```python
from build123d import *

# Parameters (mm, degrees)
F1_DEPTH = 19.05
F2_R     = 1.6880243077
F3_DEPTH = 19.05
F4_DEPTH = 19.05


with BuildPart() as f1:
    # F0 (on Front) → F1 (new body)
    with BuildSketch(Plane.XZ):
        with BuildLine():
            ThreePointArc((15.778162915, -1.0689673082), (15.8052876039, -0.5347895271), (15.8143326157, 0))
            ThreePointArc((15.8143326157, 0), (15.8010341981, 0.6484090916), (15.7611613108, 1.2957276769))
            ThreePointArc((15.7611613108, 1.2957276769), (15.0048006195, 4.9949048489), (13.3931251572, 8.4093587509))
            ThreePointArc((13.3931251572, 8.4093587509), (12.7269029213, 9.3871751934), (11.9894377321, 10.3124438882))
            ThreePointArc((11.9894377321, 10.3124438882), (9.2032072916, 12.8605634257), (5.8923688049, 14.6755955908))
            ThreePointArc((5.8923688049, 14.6755955908), (4.7786376097, 15.0750701051), (3.6381564457, 15.3901570413))
            ThreePointArc((3.6381564457, 15.3901570413), (-0.1136984162, 15.8139238884), (-3.8590721566, 15.3362537202))
            ThreePointArc((-3.8590721566, 15.3362537202), (-4.9949048489, 15.0048006195), (-6.1027769466, 14.5893532968))
            ThreePointArc((-6.1027769466, 14.5893532968), (-9.3871751934, 12.7269029213), (-12.1364787193, 10.1389841885))
            ThreePointArc((-12.1364787193, 10.1389841885), (-12.8605634257, 9.2032072916), (-13.512656971, 8.2159124668))
            ThreePointArc((-13.512656971, 8.2159124668), (-15.0750701051, 4.7786376097), (-15.778162915, 1.0689673082))
            ThreePointArc((-15.778162915, 1.0689673082), (-15.8139238884, -0.1136984162), (-15.7611613108, -1.2957276769))
            ThreePointArc((-15.7611613108, -1.2957276769), (-15.0048006195, -4.9949048489), (-13.3931251572, -8.4093587509))
            ThreePointArc((-13.3931251572, -8.4093587509), (-12.7269029213, -9.3871751934), (-11.9894377321, -10.3124438882))
            ThreePointArc((-11.9894377321, -10.3124438882), (-9.2032072916, -12.8605634257), (-5.8923688049, -14.6755955908))
            ThreePointArc((-5.8923688049, -14.6755955908), (-4.7786376097, -15.0750701051), (-3.6381564457, -15.3901570413))
            ThreePointArc((-3.6381564457, -15.3901570413), (0.1136984162, -15.8139238884), (3.8590721566, -15.3362537202))
            ThreePointArc((3.8590721566, -15.3362537202), (4.9949048489, -15.0048006195), (6.1027769466, -14.5893532968))
            ThreePointArc((6.1027769466, -14.5893532968), (9.3871751934, -12.7269029213), (12.1364787193, -10.1389841885))
            ThreePointArc((12.1364787193, -10.1389841885), (12.8605634257, -9.2032072916), (13.512656971, -8.2159124668))
            ThreePointArc((13.512656971, -8.2159124668), (15.0750701051, -4.7786376097), (15.778162915, -1.0689673082))
        make_face()
    extrude(amount=F1_DEPTH)

    # F2 (on face) → F3 (cut)
    with BuildSketch(Plane.XZ.offset(19.05)):
        Circle(F2_R)
    extrude(amount=-F3_DEPTH, mode=Mode.SUBTRACT)

    # F0 (on Front) → F4 (join)
    with BuildSketch(Plane.XZ):
        with BuildLine():
            ThreePointArc((15.7611613108, 1.2957276769), (15.8010341981, 0.6484090916), (15.8143326157, 0))
            ThreePointArc((15.8143326157, 0), (15.8052876039, -0.5347895271), (15.778162915, -1.0689673082))
            Line((15.778162915, -1.0689673082), (17.2791990232, 0.0449688409))
            Line((17.2791990232, 0.0449688409), (15.7611613108, 1.2957276769))
        make_face()
        with BuildLine():
            ThreePointArc((13.3931251572, 8.4093587509), (15.0048006195, 4.9949048489), (15.7611613108, 1.2957276769))
            Line((15.7611613108, 1.2957276769), (17.2791990232, 0.0449688409))
            Line((17.2791990232, 0.0449688409), (22.4461490806, 3.8794218687))
            Line((22.4461490806, 3.8794218687), (19.6925609503, 6.2533739679))
            Line((19.6925609503, 6.2533739679), (20.5248865096, 9.7924600538))
            Line((20.5248865096, 9.7924600538), (13.9527336374, 10.1928389138))
            Line((13.9527336374, 10.1928389138), (13.3931251572, 8.4093587509))
        make_face()
        with BuildLine():
            Line((17.2791990232, 0.0449688409), (15.778162915, -1.0689673082))
            ThreePointArc((15.778162915, -1.0689673082), (15.0750701051, -4.7786376097), (13.512656971, -8.2159124668))
            Line((13.512656971, -8.2159124668), (14.0055976804, -10.1200778007))
            Line((14.0055976804, -10.1200778007), (20.4395830263, -10.0549971802))
            Line((20.4395830263, -10.0549971802), (19.6072574669, -6.5159110943))
            Line((19.6072574669, -6.5159110943), (22.3608455972, -4.1419589951))
            Line((22.3608455972, -4.1419589951), (17.2791990232, 0.0449688409))
        make_face()
        with BuildLine():
            ThreePointArc((11.9894377321, 10.3124438882), (12.7269029213, 9.3871751934), (13.3931251572, 8.4093587509))
            Line((13.3931251572, 8.4093587509), (13.9527336374, 10.1928389138))
            Line((13.9527336374, 10.1928389138), (11.9894377321, 10.3124438882))
        make_face()
        with BuildLine():
            Line((14.0055976804, -10.1200778007), (13.512656971, -8.2159124668))
            ThreePointArc((13.512656971, -8.2159124668), (12.8605634257, -9.2032072916), (12.1364787193, -10.1389841885))
            Line((12.1364787193, -10.1389841885), (14.0055976804, -10.1200778007))
        make_face()
        with BuildLine():
            ThreePointArc((5.8923688049, 14.6755955908), (9.2032072916, 12.8605634257), (11.9894377321, 10.3124438882))
            Line((11.9894377321, 10.3124438882), (13.9527336374, 10.1928389138))
            Line((13.9527336374, 10.1928389138), (15.8790491026, 16.3320336204))
            Line((15.8790491026, 16.3320336204), (12.2559754761, 16.6340827186))
            Line((12.2559754761, 16.6340827186), (10.8491183906, 19.9864921956))
            Line((10.8491183906, 19.9864921956), (5.2967982382, 16.4473909634))
            Line((5.2967982382, 16.4473909634), (5.8923688049, 14.6755955908))
        make_face()
        with BuildLine():
            Line((14.0055976804, -10.1200778007), (12.1364787193, -10.1389841885))
            ThreePointArc((12.1364787193, -10.1389841885), (9.3871751934, -12.7269029213), (6.1027769466, -14.5893532968))
            Line((6.1027769466, -14.5893532968), (5.3823340565, -16.4195986913))
            Line((5.3823340565, -16.4195986913), (10.6257909718, -20.148749063))
            Line((10.6257909718, -20.148749063), (12.0326480574, -16.796339586))
            Line((12.0326480574, -16.796339586), (15.6557216838, -16.4942904878))
            Line((15.6557216838, -16.4942904878), (14.0055976804, -10.1200778007))
        make_face()
        with BuildLine():
            ThreePointArc((3.6381564457, 15.3901570413), (4.7786376097, 15.0750701051), (5.8923688049, 14.6755955908))
            Line((5.8923688049, 14.6755955908), (5.2967982382, 16.4473909634))
            Line((5.2967982382, 16.4473909634), (3.6381564457, 15.3901570413))
        make_face()
        with BuildLine():
            Line((5.3823340565, -16.4195986913), (6.1027769466, -14.5893532968))
            ThreePointArc((6.1027769466, -14.5893532968), (4.9949048489, -15.0048006195), (3.8590721566, -15.3362537202))
            Line((3.8590721566, -15.3362537202), (5.3823340565, -16.4195986913))
        make_face()
        with BuildLine():
            ThreePointArc((-3.8590721566, 15.3362537202), (-0.1136984162, 15.8139238884), (3.6381564457, 15.3901570413))
            Line((3.6381564457, 15.3901570413), (5.2967982382, 16.4473909634))
            Line((5.2967982382, 16.4473909634), (3.2466920765, 22.5463636346))
            Line((3.2466920765, 22.5463636346), (0.1380239354, 20.6611372425))
            Line((0.1380239354, 20.6611372425), (-2.9706442056, 22.5463636346))
            Line((-2.9706442056, 22.5463636346), (-5.3823340565, 16.4195986913))
            Line((-5.3823340565, 16.4195986913), (-3.8590721566, 15.3362537202))
        make_face()
        with BuildLine():
            Line((5.3823340565, -16.4195986913), (3.8590721566, -15.3362537202))
            ThreePointArc((3.8590721566, -15.3362537202), (0.1136984162, -15.8139238884), (-3.6381564457, -15.3901570413))
            Line((-3.6381564457, -15.3901570413), (-5.2967982382, -16.4473909634))
            Line((-5.2967982382, -16.4473909634), (-3.2466920765, -22.5463636346))
            Line((-3.2466920765, -22.5463636346), (-0.1380239354, -20.6611372425))
            Line((-0.1380239354, -20.6611372425), (2.9706442056, -22.5463636346))
            Line((2.9706442056, -22.5463636346), (5.3823340565, -16.4195986913))
        make_face()
        with BuildLine():
            ThreePointArc((-6.1027769466, 14.5893532968), (-4.9949048489, 15.0048006195), (-3.8590721566, 15.3362537202))
            Line((-3.8590721566, 15.3362537202), (-5.3823340565, 16.4195986913))
            Line((-5.3823340565, 16.4195986913), (-6.1027769466, 14.5893532968))
        make_face()
        with BuildLine():
            Line((-5.2967982382, -16.4473909634), (-3.6381564457, -15.3901570413))
            ThreePointArc((-3.6381564457, -15.3901570413), (-4.7786376097, -15.0750701051), (-5.8923688049, -14.6755955908))
            Line((-5.8923688049, -14.6755955908), (-5.2967982382, -16.4473909634))
        make_face()
        with BuildLine():
            ThreePointArc((-12.1364787193, 10.1389841885), (-9.3871751934, 12.7269029213), (-6.1027769466, 14.5893532968))
            Line((-6.1027769466, 14.5893532968), (-5.3823340565, 16.4195986913))
            Line((-5.3823340565, 16.4195986913), (-10.6257909718, 20.148749063))
            Line((-10.6257909718, 20.148749063), (-12.0326480574, 16.796339586))
            Line((-12.0326480574, 16.796339586), (-15.6557216838, 16.4942904878))
            Line((-15.6557216838, 16.4942904878), (-14.0055976804, 10.1200778007))
            Line((-14.0055976804, 10.1200778007), (-12.1364787193, 10.1389841885))
        make_face()
        with BuildLine():
            Line((-5.2967982382, -16.4473909634), (-5.8923688049, -14.6755955908))
            ThreePointArc((-5.8923688049, -14.6755955908), (-9.2032072916, -12.8605634257), (-11.9894377321, -10.3124438882))
            Line((-11.9894377321, -10.3124438882), (-13.9527336374, -10.1928389138))
            Line((-13.9527336374, -10.1928389138), (-15.8790491026, -16.3320336204))
            Line((-15.8790491026, -16.3320336204), (-12.2559754761, -16.6340827186))
            Line((-12.2559754761, -16.6340827186), (-10.8491183906, -19.9864921956))
            Line((-10.8491183906, -19.9864921956), (-5.2967982382, -16.4473909634))
        make_face()
        with BuildLine():
            ThreePointArc((-13.512656971, 8.2159124668), (-12.8605634257, 9.2032072916), (-12.1364787193, 10.1389841885))
            Line((-12.1364787193, 10.1389841885), (-14.0055976804, 10.1200778007))
            Line((-14.0055976804, 10.1200778007), (-13.512656971, 8.2159124668))
        make_face()
        with BuildLine():
            Line((-13.9527336374, -10.1928389138), (-11.9894377321, -10.3124438882))
            ThreePointArc((-11.9894377321, -10.3124438882), (-12.7269029213, -9.3871751934), (-13.3931251572, -8.4093587509))
            Line((-13.3931251572, -8.4093587509), (-13.9527336374, -10.1928389138))
        make_face()
        with BuildLine():
            ThreePointArc((-15.778162915, 1.0689673082), (-15.0750701051, 4.7786376097), (-13.512656971, 8.2159124668))
            Line((-13.512656971, 8.2159124668), (-14.0055976804, 10.1200778007))
            Line((-14.0055976804, 10.1200778007), (-20.4395830263, 10.0549971802))
            Line((-20.4395830263, 10.0549971802), (-19.6072574669, 6.5159110943))
            Line((-19.6072574669, 6.5159110943), (-22.3608455972, 4.1419589951))
            Line((-22.3608455972, 4.1419589951), (-17.2791990232, -0.0449688409))
            Line((-17.2791990232, -0.0449688409), (-15.778162915, 1.0689673082))
        make_face()
        with BuildLine():
            Line((-13.9527336374, -10.1928389138), (-13.3931251572, -8.4093587509))
            ThreePointArc((-13.3931251572, -8.4093587509), (-15.0048006195, -4.9949048489), (-15.7611613108, -1.2957276769))
            Line((-15.7611613108, -1.2957276769), (-17.2791990232, -0.0449688409))
            Line((-17.2791990232, -0.0449688409), (-22.4461490806, -3.8794218687))
            Line((-22.4461490806, -3.8794218687), (-19.6925609503, -6.2533739679))
            Line((-19.6925609503, -6.2533739679), (-20.5248865096, -9.7924600538))
            Line((-20.5248865096, -9.7924600538), (-13.9527336374, -10.1928389138))
        make_face()
        with BuildLine():
            ThreePointArc((-15.7611613108, -1.2957276769), (-15.8139238884, -0.1136984162), (-15.778162915, 1.0689673082))
            Line((-15.778162915, 1.0689673082), (-17.2791990232, -0.0449688409))
            Line((-17.2791990232, -0.0449688409), (-15.7611613108, -1.2957276769))
        make_face()
    extrude(amount=F4_DEPTH)


solid = f1.part
```
Geometry check sheet. Reference: the model listing, model coordinates, mm. A direction names the side the tool comes from. Give positions to 0.01 mm unless a question says otherwise; leave off trailing zeros. Order: outer loops, then holes, each group sorted by start corner. A loop starts at its lowest first (then second) coordinate and runs counter-clockwise, first axis right, second up.
1. Gauge pin test, flat ends, axial feed: pin 1 Ø5 at (y, z) = (-17, -14) entering from -X; pin 2 Ø5 at (y, z) = (-6.5, 12) entering from -X; pin 3 Ø10 at (x, y) = (1, -4.5) entering from +Z; pin 4 Ø2 at (x, z) = (0, 0) entering from +Y. Record the tip position at first contact, or that the pin passes through.
2. Release check for a two-part mould opening along Z. For faces 5 (the face through (11.56, -9.39, 18.29)), 6 (the face through (19.83, -9.39, 1.94)), 7 (the face through (-11.56, -9.39, -18.29)) record: pulls with the +Z half, pulls with the -Z half, needs draft (parallel to the pull), parting line crosses it, or undercut.
3. Access from +Z, -Z, +X, -X, +Y, -Y to the whole of each face (thin tool, end or side, straight path). Record for faces 1 (the face through (17.28, -9.39, 9.99)), 2 (the face through (1.714, -9.392, 21.617)), 3 (the face through (-8.11, -9.39, -18.24)), 4 (the face through (-17.28, -9.39, -9.99)).
4. Thickness scan on L1, parallel to X at y = -4.75, z = 17.5; L2, parallel to X at y = -16.75, z = -1; L3, parallel to Z at x = 0, y = -6.5. Record the ranges inside material, lowest first.
5. Section check C-C, the plane z = -12.5. Enter the section's corners in (x, y).
6. Section check B-B, the plane x = -9. Enter the section's corners in (y, z).
7. Section check A-A, the plane x = -15. Enter the section's corners in (y, z), and give its area (3 significant figures).
Values follow:
1. pin 1: stops at x = -15.88
1. pin 2: stops at x = -20.44
1. pin 3: stops at z = 22.55
1. pin 4: passes through
2. face 5: pulls with the +Z half
2. face 6: undercut
2. face 7: pulls with the -Z half
3. face 1: +X, +Y, -Y
3. face 2: +Z, +Y, -Y
3. face 3: -Z, +Y, -Y
3. face 4: -X, +Y, -Y
4. L1: x = -11.74 to -6.9, -4.96 to 4.94, 6.95 to 11.89
4. L2: x = -18.57 to -1.36, 1.36 to 18.55
4. L3: z = -20.74 to -1.69, 1.69 to 20.74
5. outline: (-14.68, -19.05) - (14.62, -19.05) - (14.62, 0) - (-14.68, 0) - close
6. outline: (-19.05, -18.81) - (0, -18.81) - (0, 18.99) - (-19.05, 18.99) - close
7. outline: (-19.05, -16.41) - (0, -16.41) - (0, -13.53) - (-19.05, -13.53) - close; (-19.05, -10.13) - (0, -10.13) - (0, 10.11) - (-19.05, 10.11) - close; (-19.05, 13.96) - (0, 13.96) - (0, 16.55) - (-19.05, 16.55) - close
7. area: 490 mm2
